For this review, take the finished solid that the model builds, in its own axes (mm). Face numbers are marked on the shaded views. Round coordinates to 2 decimals unless told otherwise and drop trailing zeros. Order: outer loops, then holes, each group sorted by start corner. A loop starts at its lowest first (then second) coordinate and runs counter-clockwise, first axis right, second up. Notation, with made-up numbers: (40, 13.25) -> (61, 13.25) arc R13 cw to (61, 35.25) -> close; hole circle Ø3 at (-14.5, 83.5). An arc over 180 degrees is marked (long way). Answer in a Markdown table with one row per item.
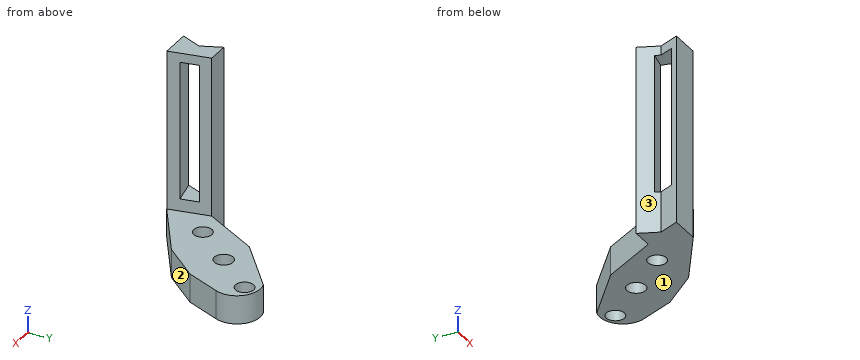
```python
from build123d import *

# Parameters (mm, degrees)
CROQUIS1_R              = 1.600993429
CROQUIS1_R_2            = 1.650918845
CROQUIS1_R_3            = 1.598160281
SALIENTE_EXTRUIR1_DEPTH = 5
SALIENTE_EXTRUIR2_DEPTH = 28
CROQUIS3_W              = 24.234712775
CROQUIS3_H              = 3.1
CORTAR_EXTRUIR2_DEPTH   = 35


with BuildPart() as part:
    # Croquis1 → Saliente-Extruir1 (new body)
    with BuildSketch(Plane.XY):
        with BuildLine():
            Line((-19.813726886, 27.408212729), (-22.344749079, 27.408212729))
            Line((-22.344749079, 27.408212729), (-20.84194462, 23.881480403))
            Line((-20.84194462, 23.881480403), (-22.344749079, 20.354748078))
            Line((-22.344749079, 20.354748078), (-19.813726886, 20.354748078))
            Line((-19.813726886, 20.354748078), (-17.089167092, 20.354748078))
            ThreePointArc((-17.089167092, 20.354748078), (-17.073233268, 20.346247985), (-17.05726125, 20.337819881))
            Line((-17.05726125, 20.337819881), (-6.693946802, 26.960720035))
            Line((-6.693946802, 26.960720035), (-1.55164568, 33.089075871))
            Line((-1.55164568, 33.089075871), (0.94121729, 39.089722795))
            ThreePointArc((0.94121729, 39.089722795), (0.14668389, 43.447470603), (-4.153529562, 44.510209303))
            Line((-4.153529562, 44.510209303), (-13.213359782, 36.992537931))
            Line((-13.213359782, 36.992537931), (-18.553173623, 27.408212729))
            Line((-18.553173623, 27.408212729), (-19.813726886, 27.408212729))
        make_face()
        with Locations((-2.081556076, 42.38660259)):
            Circle(CROQUIS1_R, mode=Mode.SUBTRACT)
        with Locations((-7.865918923, 35.491404278)):
            Circle(CROQUIS1_R_2, mode=Mode.SUBTRACT)
        with Locations((-13.649232709, 28.598160609)):
            Circle(CROQUIS1_R_3, mode=Mode.SUBTRACT)
    extrude(amount=SALIENTE_EXTRUIR1_DEPTH)

    # Croquis2 → Saliente-Extruir2 (add)
    with BuildSketch(Plane.XY.offset(5)):
        Polygon((-22.344749079, 20.354748078), (-17.089167092, 20.354748078), (-18.553173623, 27.408212729), (-22.344749079, 27.408212729), (-20.84194462, 23.881480403), align=None)
    extrude(amount=SALIENTE_EXTRUIR2_DEPTH)

    # Croquis3 → Cortar-Extruir2 (cut)
    with BuildSketch(Plane(origin=(-12.33305174, -2.559829698, 0), x_dir=(0, 0, -1), z_dir=(0.9791316303558096, 0.2032270908042881, 0))):
        with Locations((-19.260916646, 27.056755515)):
            Rectangle(CROQUIS3_W, CROQUIS3_H)
    extrude(amount=-CORTAR_EXTRUIR2_DEPTH, mode=Mode.SUBTRACT)


solid = part.part
```
Q1. Take a section at C-C, the plane x = -5.75. Write out the cut boundary in (y, z).
Answer key:
| item | result |
|---|---|
| outline | (28.09, 0) -> (43.19, 0) -> (43.19, 5) -> (28.09, 5) -> close |
Q2. Take a section at B-B, the plane x = -12.5. Write out the cut boundary in (y, z), then the cut area to 3 significant figures.
Answer key:
| item | result |
|---|---|
| outline | (23.25, 0) -> (27.49, 0) -> (27.49, 5) -> (23.25, 5) -> close; (29.71, 0) -> (37.58, 0) -> (37.58, 5) -> (29.71, 5) -> close |
| area | 60.6 mm^2 |
Q3. To check wall thickness, follow probe 1 along Z at (x, y) = (-9, 38); probe 2 along Y at (x, z) = (-20, 10); probe 3 along Y at (x, z) = (-18, 12). State the ranges of each line that lie inside material, in increasing order.
Answer key:
| item | result |
|---|---|
| probe 1 | z = 0 to 5 |
| probe 2 | y = 20.35 to 21.9, 25.07 to 27.41 |
| probe 3 | y = 20.35 to 22.31 |
Q4. Clearance check with flat-ended pins moving along their axes: pin 1 Ø12 at (y, z) = (41, 9) entering from +X; pin 2 Ø1.6 at (x, z) = (-20, 24) entering from -Y; pin 3 Ø3 at (x, z) = (-21, 19.5) entering from +Y; pin 4 Ø10 at (x, y) = (-13.5, 35) entering from +Z. State where each tip first meets the part, or that it passes through.
Answer key:
| item | result |
|---|---|
| pin 1 | stops at x = 1.25 |
| pin 2 | stops at y = 20.35 |
| pin 3 | stops at y = 27.41 |
| pin 4 | stops at z = 5 |
Q5. The part is to be moulded in two halves that separate along Y. For the marked faces 1, 2 and 3, say which applies: +Y half, -Y half, draft (parallel to the pull), parting line (faces both ways), or undercut.
Answer key:
| item | result |
|---|---|
| face 1 | draft |
| face 2 | -Y half |
| face 3 | undercut |
Q6. Take a section at A-A, the plane z = 24.5. Write out the cut boundary in (x, y).
Answer key:
| item | result |
|---|---|
| outline | (-22.34, 20.35) -> (-17.09, 20.35) -> (-17.52, 22.41) -> (-21.85, 21.52) -> close; (-22.34, 27.41) -> (-21.24, 24.81) -> (-18.15, 25.45) -> (-18.55, 27.41) -> close |
